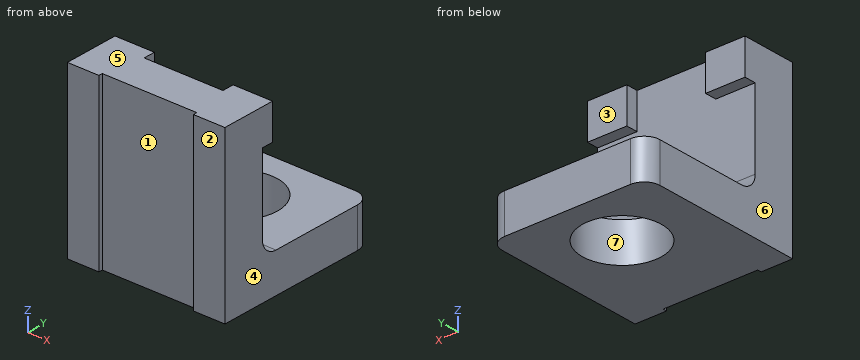
Autodesk Inventor part; units mm, degrees
ref_plane "YZ Plane" through (0, 0, 0) normal (1, 0, 0) x (0, 1, 0)
ref_plane "XZ Plane" through (0, 0, 0) normal (0, 1, 0) x (-1, 0, 0)
ref_plane "XY Plane" through (0, 0, 0) normal (0, 0, 1) x (1, 0, 0)
sketch "Sketch4" plane through (0, 0, 0) normal (0, 0, 1) x (1, 0, 0)
  circle A0 centre (0, 0) radius 31.75
  line L0 (-63.5, -50.8) -> (63.5, -50.8) construction
  line L1 (63.5, -50.8) -> (63.5, 50.8)
  line L2 (63.5, 50.8) -> (-63.5, 50.8)
  line L3 (-63.5, 50.8) -> (-63.5, -50.8)
  line L4 (-63.5, -50.8) -> (63.5, 50.8) construction
  line L5 (63.5, -50.8) -> (-63.5, 50.8) construction
  line L6 (-63.5, -50.8) -> (63.5, -50.8) construction
  line L7 (63.5, -50.8) -> (63.5, -85.725)
  line L8 (63.5, -85.725) -> (-63.5, -85.725)
  line L9 (-63.5, -85.725) -> (-63.5, -50.8)
  dimension "d2" = 127
  dimension "d3" = 101.6
  dimension "d4" = 63.5
  dimension "d5" = 136.525
extrude "Extrusion1" add sketch "Sketch4" along normal blind 31.75
sketch "Sketch5" plane through (0, 0, 31.75) normal (0, 0, 1) x (1, 0, 0)
  line L0 (-63.5, 50.8) -> (-63.5, -85.725)
  line L1 (-63.5, -85.725) -> (63.5, -85.725)
  line L2 (63.5, -85.725) -> (63.5, -41.275)
  line L3 (63.5, -41.275) -> (-63.5, -41.275)
  line L4 (-63.5, -41.275) -> (-63.5, -85.725)
  line L5 (63.5, -85.725) -> (63.5, 50.8)
  line L6 (-63.5, -41.275) -> (63.5, -41.275)
  line L7 (63.5, -41.275) -> (63.5, -50.8)
  line L8 (63.5, -50.8) -> (-63.5, -50.8)
  line L9 (-63.5, -50.8) -> (-63.5, -41.275)
  point P0 (0, 0)
  point P1 (-63.5, -50.8)
  dimension "d8" = 44.45
  dimension "d9" = 9.525
extrude "Extrusion2" add sketch "Sketch5" along normal blind 104.775 contours L8 L2 L1 L0
sketch "Sketch6" plane through (0, 0, 136.525) normal (0, 0, 1) x (1, 0, 0)
  line L0 (-63.5, -85.725) -> (63.5, -85.725)
  line L1 (-38.1, -85.725) -> (38.1, -85.725)
  line L2 (38.1, -85.725) -> (38.1, -82.55)
  line L3 (38.1, -82.55) -> (-38.1, -82.55)
  line L4 (-38.1, -82.55) -> (-38.1, -85.725)
  line L5 (-63.5, -50.8) -> (-63.5, -85.725)
  point P0 (0, 0)
  dimension "d12" = 3.175
  dimension "d13" = 25.4
  dimension "d14" = 76.2
extrude "Extrusion3" cut sketch "Sketch6" against normal through all
sketch "Sketch7" plane through (-63.5, -50.8, 31.75) normal (0, 1, 0) x (1, 0, 0)
  line L0 (127, -104.775) -> (0, -104.775)
  line L1 (0, -104.775) -> (31.75, -104.775)
  line L2 (31.75, -104.775) -> (31.75, -76.2)
  line L3 (31.75, -76.2) -> (0, -76.2)
  line L4 (0, -76.2) -> (0, -104.775)
  line L5 (127, 31.75) -> (127, -104.775)
  line L6 (95.25, -104.775) -> (127, -104.775)
  line L7 (127, -104.775) -> (127, -76.2)
  line L8 (127, -76.2) -> (95.25, -76.2)
  line L9 (95.25, -76.2) -> (95.25, -104.775)
  line L10 (0, 0) -> (127, 0)
  point P0 (63.5, 31.75)
  dimension "d17" = 63.5
  dimension "d18" = 76.2
extrude "Extrusion4" add sketch "Sketch7" along normal blind 9.525
fillet "Fillet1" radius 12.7 3 edges at (63.5, 50.8, 15.875) (-63.5, 50.8, 15.875) (0, -50.8, 31.75)
properties part number "TubeMount"
Here's how the part is built. I have some questions about the finished solid (model axes, mm). Face numbers are marked on the shaded views. A direction names the side the tool comes from. Give positions to 0.01 mm unless a question says otherwise; leave off trailing zeros. Order: outer loops, then holes, each group sorted by start corner. A loop starts at its lowest first (then second) coordinate and runs counter-clockwise, first axis right, second up. Notation, with made-up numbers: (6.5, 57.25) -> (55.5, 57.25) arc R15 cw to (55.5, 70.25) -> close; hole circle Ø5 at (-33, 27.5). An arc over 180 degrees is marked (long way). Use a Markdown table: item, result. Add a question column.
Item 1: If we mould it in two halves opening along X, with no side actions, what happens to the marked faces 4, 5, 6 and 7? For each: pulls with the +X half, pulls with the -X half, needs draft (parallel to the pull), parting line crosses it, or undercut.
Item 2: Imagine slicing it at A-A on x = 0. Please give me the cut outline in (y, z) (3 decimals).
Item 3: Imagine slicing it at C-C on y = 0. Please give me the cut outline in (x, z).
Item 4: For the marked faces 1, 2 and 3, which set-ups out of +Z, -Z, +X, -X, +Y, -Y let a thin tool reach every point of the face, with its end or its side?
Item 5: Imagine slicing it at B-B on z = 28. Please give me the cut outline in (x, y) (3 decimals), plus the area to 3 significant figures.
Item 6: Imagine slicing it at D-D on z = 113. Please give me the cut outline in (x, y) (3 decimals).
Item 7: I need wall thicknesses on line 1 (Y direction, x = 0, z = 9.5); line 2 (Y direction, x = -2.5, z = 79); line 3 (Y direction, x = 15, z = 18.5). Which ranges of each line are inside material? Lowest first, please.
Item 8: Will these pins go through, and if not, where does the flat tip stop? pin 1 (4 mm diameter, centred on x = -3, z = 79.5, fed in from -Y); pin 2 (23 mm diameter, centred on x = 51.5, z = 128.5, fed in from +Y) (3 decimals); pin 3 (5 mm diameter, centred on x = -34.5, z = 85.5, fed in from +Y).
Data:
| question | item | result |
|---|---|---|
| 1 | face 4 | pulls with the +X half |
| 1 | face 5 | needs draft |
| 1 | face 6 | pulls with the -X half |
| 1 | face 7 | undercut |
| 2 | outline | (-82.55, 0) -> (-31.75, 0) -> (-31.75, 31.75) -> (-38.1, 31.75) arc R12.7 cw to (-50.8, 44.45) -> (-50.8, 136.525) -> (-82.55, 136.525) -> close; (31.75, 0) -> (50.8, 0) -> (50.8, 31.75) -> (31.75, 31.75) -> close |
| 3 | outline | (-63.5, 0) -> (-31.75, 0) -> (-31.75, 31.75) -> (-63.5, 31.75) -> close; (31.75, 0) -> (63.5, 0) -> (63.5, 31.75) -> (31.75, 31.75) -> close |
| 4 | face 1 | +Z, -Z, -Y |
| 4 | face 2 | +Z, -Z, +X, -X, -Y |
| 4 | face 3 | +Z, +X, -X, +Y |
| 5 | outline | (-63.5, -85.725) -> (-38.1, -85.725) -> (-38.1, -82.55) -> (38.1, -82.55) -> (38.1, -85.725) -> (63.5, -85.725) -> (63.5, 38.1) arc R12.7 ccw to (50.8, 50.8) -> (-50.8, 50.8) arc R12.7 ccw to (-63.5, 38.1) -> close; hole circle Ø63.5 at (0, 0) |
| 5 | area | 13,900 mm² |
| 6 | outline | (-63.5, -85.725) -> (-38.1, -85.725) -> (-38.1, -82.55) -> (38.1, -82.55) -> (38.1, -85.725) -> (63.5, -85.725) -> (63.5, -41.275) -> (31.75, -41.275) -> (31.75, -50.8) -> (-31.75, -50.8) -> (-31.75, -41.275) -> (-63.5, -41.275) -> close |
| 7 | line 1 | y = -82.55 to -31.75, 31.75 to 50.8 |
| 7 | line 2 | y = -82.55 to -50.8 |
| 7 | line 3 | y = -82.55 to -27.98, 27.98 to 50.8 |
| 8 | pin 1 | stops at y = -82.55 |
| 8 | pin 2 | stops at y = -41.275 |
| 8 | pin 3 | stops at y = -50.8 |
